Geometry: final body of the model. Coordinates: model frame, mm. Coordinates: 2 decimals unless noted, no trailing zeros. Loops run counter-clockwise (first coordinate to the right, second up) from the corner with the lowest first, then second, coordinate; pieces in that order, holes last. Notation, with made-up numbers: (-18.5, 18) -> (2.5, 18) arc R11 ccw to (2.5, 34) -> close; hole circle Ø9 at (34, -23.5). An arc over 180 degrees is marked (long way). One line per item, written item: value. Start each with the question number.
Item 1: Ray query, probe 1 along Y at (x, z) = (115, 2.25); probe 2 along Y at (x, z) = (-115, 0.9); probe 3 along Y at (x, z) = (78, 1.85). Return the intervals inside material, ascending. Write a range as from..to.
Item 2: Section query A-A on z = 2. Return loops of the section in (x, y), then the cut area to 3 significant figures.
Item 3: Contact query for flat-ended pins moving along their axis: pin 1 Ø6.5 at (x, y) = (-115, 0) entering from -Z; pin 2 Ø2 at (y, z) = (78, 2.5) entering from -X; pin 3 Ø2 at (y, z) = (73, 2) entering from -X. Output: stop coordinate, or through.
Item 4: Section query B-B on y = 0. Return loops of the section in (x, z).
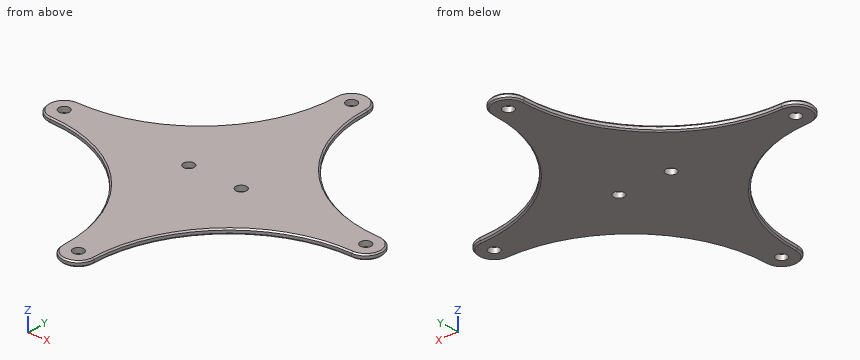
from build123d import *

# Parameters (mm, degrees)
IZIM1_R                     = 132.5
IZIM1_R_2                   = 4
Y_KSEKLIK_EKSTR_ZYON1_DEPTH = 4
SKETCH1_R                   = 147.896519427
CUT_EXTRUDE2_DEPTH          = 10
CHAMFER1_SIZE               = 1


with BuildPart() as part:
    # Çizim1 → Yükseklik-Ekstrüzyon1 (new body)
    with BuildSketch(Plane.XY):
        Circle(IZIM1_R)
        with Locations((0, 115)):
            Circle(IZIM1_R_2, mode=Mode.SUBTRACT)
        with Locations((115, 0)):
            Circle(IZIM1_R_2, mode=Mode.SUBTRACT)
        with Locations((0, -115)):
            Circle(IZIM1_R_2, mode=Mode.SUBTRACT)
        with Locations((-115, 0)):
            Circle(IZIM1_R_2, mode=Mode.SUBTRACT)
        with Locations((-20, 0)):
            Circle(IZIM1_R_2, mode=Mode.SUBTRACT)
        with Locations((20, 0)):
            Circle(IZIM1_R_2, mode=Mode.SUBTRACT)
    extrude(amount=Y_KSEKLIK_EKSTR_ZYON1_DEPTH)

    # Sketch1 → Cut-Extrude2 (cut)
    with BuildSketch(Plane.XY.offset(4)):
        Circle(SKETCH1_R)
        with BuildLine():
            ThreePointArc((12, 115), (0, 127), (-12, 115))
            ThreePointArc((-12, 115), (-42.168001538, 42.168001538), (-115, 12))
            ThreePointArc((-115, 12), (-127, 0), (-115, -12))
            ThreePointArc((-115, -12), (-42.168001538, -42.168001538), (-12, -115))
            ThreePointArc((-12, -115), (0, -127), (12, -115))
            ThreePointArc((12, -115), (42.168001538, -42.168001538), (115, -12))
            ThreePointArc((115, -12), (127, 0), (115, 12))
            ThreePointArc((115, 12), (42.168001538, 42.168001538), (12, 115))
        make_face(mode=Mode.SUBTRACT)
    extrude(amount=-CUT_EXTRUDE2_DEPTH, mode=Mode.SUBTRACT)

    # Chamfer1
    chamfer1_edges = [part.edges().sort_by_distance(p)[0] for p in [
        (127, 0, 0),
        (42.168001538, 42.168001538, 0),
        (0, 127, 0),
        (-42.168001538, 42.168001538, 0),
        (-127, 0, 0),
        (-42.168001538, -42.168001538, 0),
        (0, -127, 0),
        (42.168001538, -42.168001538, 0),
        (-42.168001538, -42.168001538, 4),
        (-127, 0, 4),
        (0, 127, 4),
        (42.168001538, 42.168001538, 4),
        (127, 0, 4),
        (42.168001538, -42.168001538, 4),
        (0, -127, 4),
        (-42.168001538, 42.168001538, 4),
    ]]
    chamfer(chamfer1_edges, length=CHAMFER1_SIZE)


solid = part.part
Reply:
1. probe 1: y = -12..-4, 4..12
1. probe 2: y = -11.9..-4, 4..11.9
1. probe 3: y = -18.88..18.88
2. outline: (-115, -12) arc R103 cw to (-12, -115) arc R12 ccw to (12, -115) arc R103 cw to (115, -12) arc R12 ccw to (115, 12) arc R103 cw to (12, 115) arc R12 ccw to (-12, 115) arc R103 cw to (-115, 12) arc R12 ccw to start; hole circle Ø8 at (-115, 0); hole circle Ø8 at (-20, 0); hole circle Ø8 at (0, -115); hole circle Ø8 at (0, 115); hole circle Ø8 at (20, 0); hole circle Ø8 at (115, 0)
2. area: 20,200 mm²
3. pin 1: passes through
3. pin 2: stops at x = -19.27
3. pin 3: stops at x = -21.41
4. outline: (-127, 1) -> (-126, 0) -> (-119, 0) -> (-119, 4) -> (-126, 4) -> (-127, 3) -> close; (-111, 0) -> (-24, 0) -> (-24, 4) -> (-111, 4) -> close; (-16, 0) -> (16, 0) -> (16, 4) -> (-16, 4) -> close; (24, 0) -> (111, 0) -> (111, 4) -> (24, 4) -> close; (119, 0) -> (126, 0) -> (127, 1) -> (127, 3) -> (126, 4) -> (119, 4) -> close
